Job drawing, mm, ordinate dimensions from the low corner. One solid piece. A direction names the side the tool comes from. Round coordinates to 2 decimals unless told otherwise and drop trailing zeros. Write each loop counter-clockwise with the first axis right and the second up, starting at its lowest first coordinate (ties: lowest second). Pieces come first, ordered by that corner, then holes.
1) Wall check: probe 1 along X at (y, z) = (23, 32.5); probe 2 along Z at (x, y) = (18, 33); probe 3 along Y at (x, z) = (19.5, 27). Give the ranges that are in metal, low to high.
2) Saw through at B-B (x = 10). Write the cut outline in (y, z).
3) Which spindle directions (+Z, -Z, +X, -X, +Y, -Y) get a long thin tool onto all of the face, cutting with end or side? Do the marked faces 1, 2, 3 and 4. Say none if no direction does.
4) Saw through at C-C (z = 45.5). Write the cut outline in (x, y), plus the area to 3 significant figures.
5) Flat gauge pins, fed straight in: pin 1 (4 mm diameter, centred on x = 3.5, y = 9.5, fed in from -Z); pin 2 (13 mm diameter, centred on x = 12, y = 29, fed in from +Z) (1 decimal); pin 3 (4 mm diameter, centred on x = 9.5, z = 45, fed in from +Y); pin 4 (5 mm diameter, centred on y = 34.5, z = 15.5, fed in from +X). Where does each tip first touch, or does it go through?
6) Saw through at A-A (x = 22.5). Write the cut outline in (y, z).
7) Saw through at D-D (y = 16.5). Write the cut outline in (x, z), plus the area to 3 significant figures.
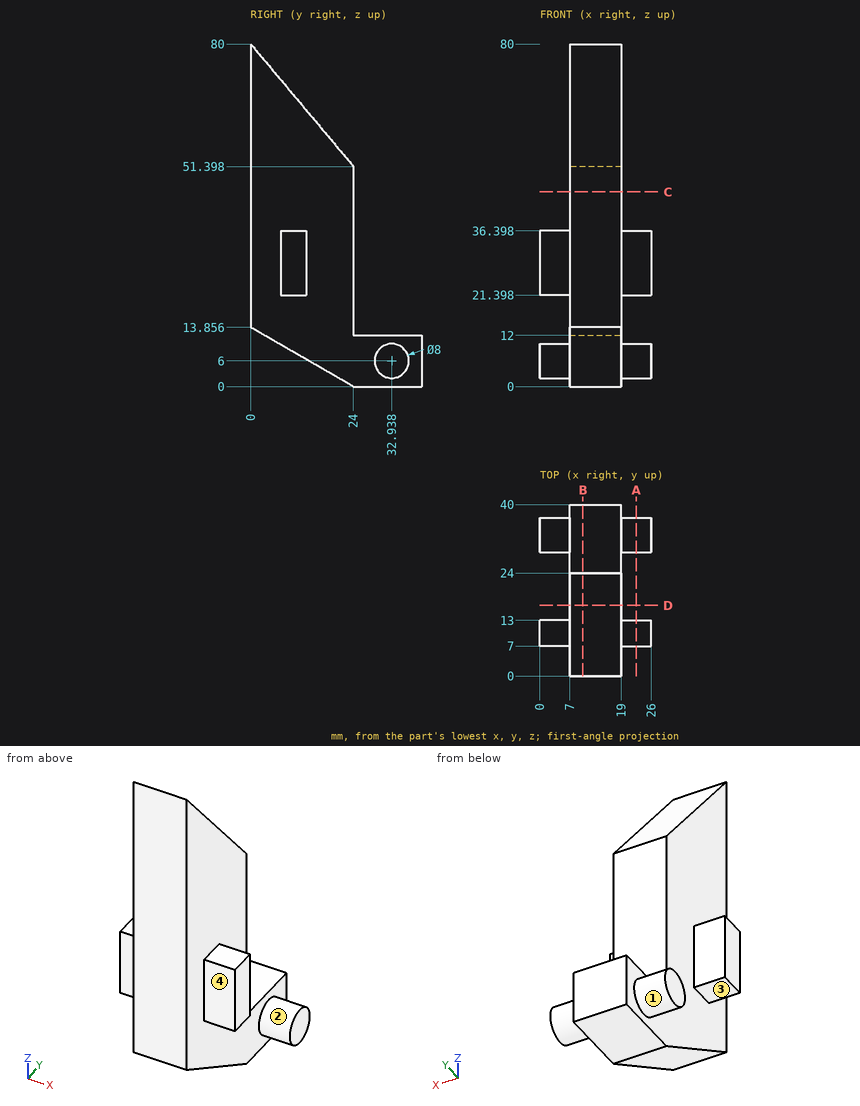
Evaluation:
1. probe 1: x = 7 to 19
1. probe 2: z = 0 to 12
1. probe 3: y = 7 to 13
2. outline: (0, 13.86) - (24, 0) - (40, 0) - (40, 12) - (24, 12) - (24, 51.4) - (0, 80) - close
3. face 1: -X
3. face 2: +X
3. face 3: -Z, -X, +Y, -Y
3. face 4: +Z, -Z, +X, -Y
4. outline: (7, 0) - (19, 0) - (19, 24) - (7, 24) - close
4. area: 288 mm2
5. pin 1: stops at z = 21.4
5. pin 2: stops at z = 53.2
5. pin 3: stops at y = 24
5. pin 4: passes through
6. outline: (7, 21.4) - (13, 21.4) - (13, 36.4) - (7, 36.4) - close; circle Ø8 at (32.94, 6)
7. outline: (7, 4.33) - (19, 4.33) - (19, 60.34) - (7, 60.34) - close
7. area: 672 mm2
